from build123d import *

# Parameters (mm, degrees)
SKETCH_W     = 166
SKETCH_H     = 134
SKETCH_W_2   = 80
SKETCH_H_2   = 20
PAD_DEPTH    = 50
POCKET_DEPTH = 166.001
SKETCH002_W  = 30
SKETCH002_H  = 130
PAD001_DEPTH = 2
FILLET_R     = 0.5


with BuildPart() as part:
    # Sketch → Pad (new body)
    with BuildSketch(Plane.XY):
        Rectangle(SKETCH_W, SKETCH_H)
        with Locations((-41, -55)):
            Rectangle(SKETCH_W_2, SKETCH_H_2, mode=Mode.SUBTRACT)
        with Locations((-41, -33)):
            Rectangle(SKETCH_W_2, SKETCH_H_2, mode=Mode.SUBTRACT)
        with Locations((-41, -11)):
            Rectangle(SKETCH_W_2, SKETCH_H_2, mode=Mode.SUBTRACT)
        with Locations((-41, 11)):
            Rectangle(SKETCH_W_2, SKETCH_H_2, mode=Mode.SUBTRACT)
        with Locations((-41, 33)):
            Rectangle(SKETCH_W_2, SKETCH_H_2, mode=Mode.SUBTRACT)
        with Locations((-41, 55)):
            Rectangle(SKETCH_W_2, SKETCH_H_2, mode=Mode.SUBTRACT)
        with Locations((41, 55)):
            Rectangle(SKETCH_W_2, SKETCH_H_2, mode=Mode.SUBTRACT)
        with Locations((41, 33)):
            Rectangle(SKETCH_W_2, SKETCH_H_2, mode=Mode.SUBTRACT)
        with Locations((41, 11)):
            Rectangle(SKETCH_W_2, SKETCH_H_2, mode=Mode.SUBTRACT)
        with Locations((41, -11)):
            Rectangle(SKETCH_W_2, SKETCH_H_2, mode=Mode.SUBTRACT)
        with Locations((41, -33)):
            Rectangle(SKETCH_W_2, SKETCH_H_2, mode=Mode.SUBTRACT)
        with Locations((41, -55)):
            Rectangle(SKETCH_W_2, SKETCH_H_2, mode=Mode.SUBTRACT)
    extrude(amount=PAD_DEPTH)

    # Sketch001 (on Face2 of Pad) → Pocket (cut, through all)
    with BuildSketch(Plane.YZ.offset(83)):
        Polygon((-72, 40), (72, 50), (72, 60), (-72, 60), align=None)
    extrude(amount=-POCKET_DEPTH, mode=Mode.SUBTRACT)

    # Sketch002 (on Face2 of Pocket) → Pad001 (join)
    with BuildSketch(Plane(origin=(0, 0, 0), x_dir=(1, 0, 0), z_dir=(0, 0, -1))):
        with Locations((-41, 0)):
            Rectangle(SKETCH002_W, SKETCH002_H)
        with Locations((41, 0)):
            Rectangle(SKETCH002_W, SKETCH002_H)
    extrude(amount=-PAD001_DEPTH)

    # Fillet
    fillet_edges = [part.edges().sort_by_distance(p)[0] for p in [
        (83, 0, 45),
        (0, 67, 49.652778),
        (-83, 0, 45),
        (0, -67, 40.347222),
        (-41, -65, 40.486111),
        (-81, -55, 41.180556),
        (-41, -45, 41.875),
        (-1, -55, 41.180556),
        (-81, -33, 42.708333),
        (-41, -23, 43.402778),
        (-1, -33, 42.708333),
        (-41, -43, 42.013889),
        (-81, -11, 44.236111),
        (-41, -1, 44.930556),
        (-1, -11, 44.236111),
        (-41, -21, 43.541667),
        (-81, 11, 45.763889),
        (-41, 21, 46.458333),
        (-1, 11, 45.763889),
        (-41, 1, 45.069444),
        (-81, 33, 47.291667),
        (-41, 43, 47.986111),
        (-1, 33, 47.291667),
        (-41, 23, 46.597222),
        (-81, 55, 48.819444),
        (-41, 65, 49.513889),
        (-1, 55, 48.819444),
        (-41, 45, 48.125),
        (81, -55, 41.180556),
        (41, -65, 40.486111),
        (1, -55, 41.180556),
        (41, -45, 41.875),
        (81, -33, 42.708333),
        (41, -43, 42.013889),
        (1, -33, 42.708333),
        (41, -23, 43.402778),
        (81, -11, 44.236111),
        (41, -21, 43.541667),
        (1, -11, 44.236111),
        (41, -1, 44.930556),
        (81, 11, 45.763889),
        (41, 1, 45.069444),
        (1, 11, 45.763889),
        (41, 21, 46.458333),
        (81, 33, 47.291667),
        (41, 23, 46.597222),
        (1, 33, 47.291667),
        (41, 43, 47.986111),
        (81, 55, 48.819444),
        (41, 45, 48.125),
        (1, 55, 48.819444),
        (41, 65, 49.513889),
        (-83, -67, 20.173611),
        (83, 67, 24.826389),
        (-81, 65, 24.756944),
        (83, -67, 20.173611),
    ]]
    fillet(fillet_edges, radius=FILLET_R)


solid = part.part
The listing builds one solid part. Answer for the finished solid, in the listing's coordinates (mm). A direction names the side the tool comes from. Round coordinates to 2 decimals unless told otherwise and drop trailing zeros. Use a Markdown table: item, result. Add a question column.
1. A tool of negligible diameter and unlimited length cuts with its end or side. For faces 1 (the face through (-81, -55, 20)), 2 (the face through (83, -1, 24)), 3 (the face through (-42, -65, 20)), from which of +Z, -Z, +X, -X, +Y, -Y can it reach the whole face along a straight path? Write none if from no direction.
2. A flat-ended cylindrical pin translates along its axis: P1, Ø10, axis at x = -40.5, y = 53.5, coming from the +Z side. Find the tip coordinate at first contact, or state that the pin passes through.
3. The part is cut by section A-A (z = 11). Give the number of separate pieces and of enclosed holes in the cut face, and give its area (3 significant figures).
4. Consider line 1 (X direction, y = -7, z = 20); line 2 (Y direction, x = -16, z = 43); line 3 (Y direction, x = -41, z = 40.5). Determine where each line is inside the solid, lowest interval first.
5. For a pull along Y with two mould halves and no side action, classify faces 4 (the face through (36, -1, 0)), 5 (the face through (81, 11, 23)), 6 (the face through (-82.85, -0.71, 44.81)) as +Y half, -Y half, draft (parallel to the pull), parting line (faces both ways), or undercut.
Reported:
| question | item | result |
|---|---|---|
| 1 | face 1 | +Z, -Z |
| 1 | face 2 | +Z, -Z, +X, +Y, -Y |
| 1 | face 3 | +Z |
| 2 | P1 | z = 2 |
| 3 | separate pieces | 1 |
| 3 | enclosed holes | 12 |
| 3 | area | 3,040 mm^2 |
| 4 | line 1 | -83 to -81, -1 to 1, 81 to 83 |
| 4 | line 2 | -23 to -21, -1 to 1, 21 to 23, 43 to 45, 65 to 67 |
| 4 | line 3 | -45 to -43, -23 to -21, -1 to 1, 21 to 23, 43 to 45, 65 to 67 |
| 5 | face 4 | draft |
| 5 | face 5 | undercut |
| 5 | face 6 | -Y half |
